Study the drawing (mm; zero at the part's minimum x, y, z) and answer. A direction names the side the tool comes from. Give positions to 0.01 mm unless a question says otherwise; leave off trailing zeros. Order: outer loops, then holes, each group sorted by start corner. A loop starts at its lowest first (then second) coordinate and runs counter-clockwise, first axis right, second up.
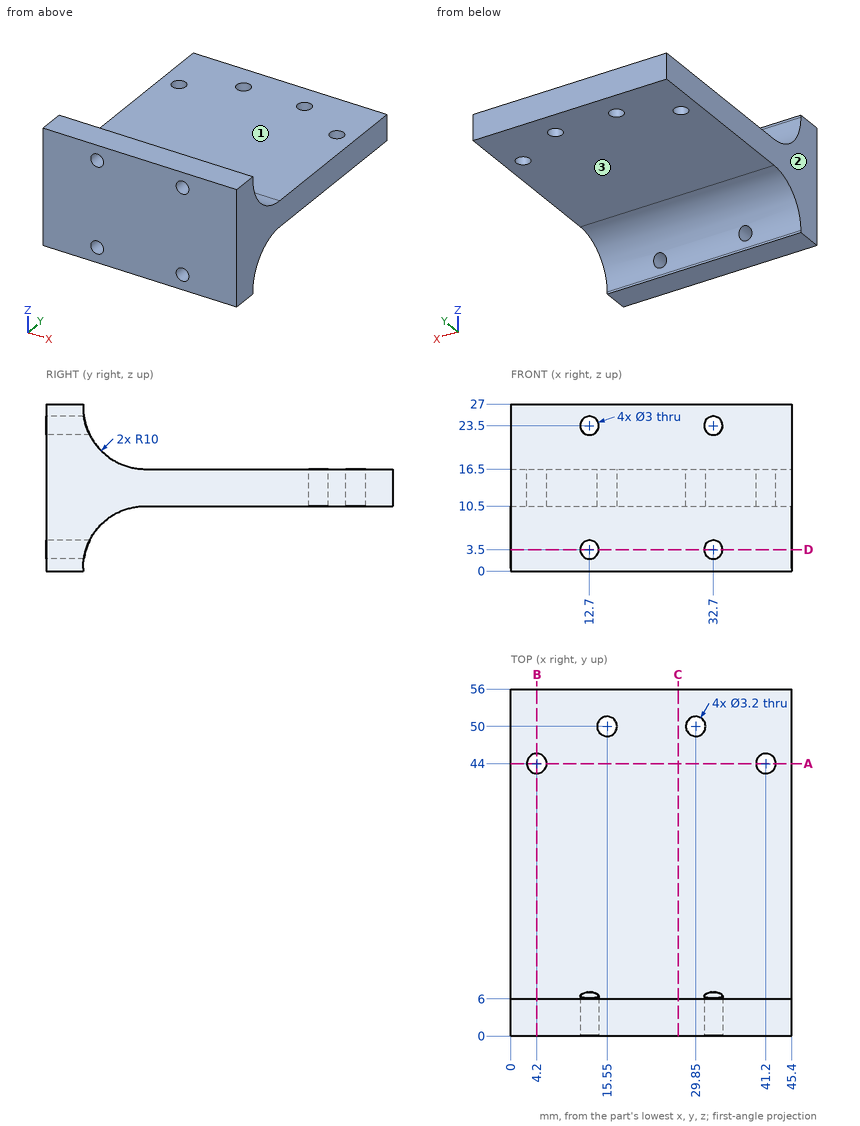
1) Find section D-D (z = 3.5). Write down the section's boundary in (x, y).
Geometry says:
outline: (0, 0) - (11.2, 0) - (11.2, 6.46) - (0, 6.46) - close; (14.2, 0) - (31.2, 0) - (31.2, 6.46) - (14.2, 6.46) - close; (34.2, 0) - (45.4, 0) - (45.4, 6.46) - (34.2, 6.46) - close
2) Find section B-B (x = 4.2). Write down the section's boundary in (y, z), then the cut area to 3 significant figures.
Geometry says:
outline: (0, 0) - (6, 0) - (6, 0.5) arc R10 cw to (16, 10.5) - (42.4, 10.5) - (42.4, 16.5) - (16, 16.5) arc R10 cw to (6, 26.5) - (6, 27) - (0, 27) - close; (45.6, 10.5) - (56, 10.5) - (56, 16.5) - (45.6, 16.5) - close
area: 486 mm2
3) Given P1, Ø20, axis at x = 32.5, y = 27, coming from the -Z side; P2, Ø5, axis at x = 4.2, y = 44, coming from the +Z side; P3, Ø5, axis at x = 32.7, z = 3.5, coming from the +Y side, each flat-ended and moving along its own axis, determine where each tip first touches the part or whether it passes through.
Geometry says:
P1: stops at z = 10.5
P2: stops at z = 16.5
P3: stops at y = 7.65
4) Find section A-A (y = 44). Write down the section's boundary in (x, z).
Geometry says:
outline: (0, 10.5) - (2.6, 10.5) - (2.6, 16.5) - (0, 16.5) - close; (5.8, 10.5) - (39.6, 10.5) - (39.6, 16.5) - (5.8, 16.5) - close; (42.8, 10.5) - (45.4, 10.5) - (45.4, 16.5) - (42.8, 16.5) - close
5) A tool of negligible diameter and unlimited length cuts with its end or side. For the marked faces 1, 2 and 3, from which of +Z, -Z, +X, -X, +Y, -Y can it reach the whole face along a straight path? Write none if from no direction.
Geometry says:
face 1: +Z, +X, -X, +Y
face 2: +Z, -Z, -X, +Y, -Y
face 3: -Z, +X, -X, +Y
6) Find section C-C (x = 27). Write down the section's boundary in (y, z).
Geometry says:
outline: (0, 0) - (6, 0) - (6, 0.5) arc R10 cw to (16, 10.5) - (56, 10.5) - (56, 16.5) - (16, 16.5) arc R10 cw to (6, 26.5) - (6, 27) - (0, 27) - close
7) Straight lines are drawn through the part: probe 1 along X at (y, z) = (2.75, 23.5); probe 2 along Z at (x, y) = (11, 30); probe 3 along Y at (x, z) = (29.5, 15.75). For each, find the intervals that lie inside material, in ascending order.
Geometry says:
probe 1: x = 0 to 11.2, 14.2 to 31.2, 34.2 to 45.4
probe 2: z = 10.5 to 16.5
probe 3: y = 0 to 48.44, 51.56 to 56
